Geometry check sheet. Reference: the model listing, model coordinates, mm. Face numbers are marked on the shaded views. A direction names the side the tool comes from. Round coordinates to 2 decimals unless told otherwise and drop trailing zeros. Loops run counter-clockwise (first coordinate to the right, second up) from the corner with the lowest first, then second, coordinate; pieces in that order, holes last.
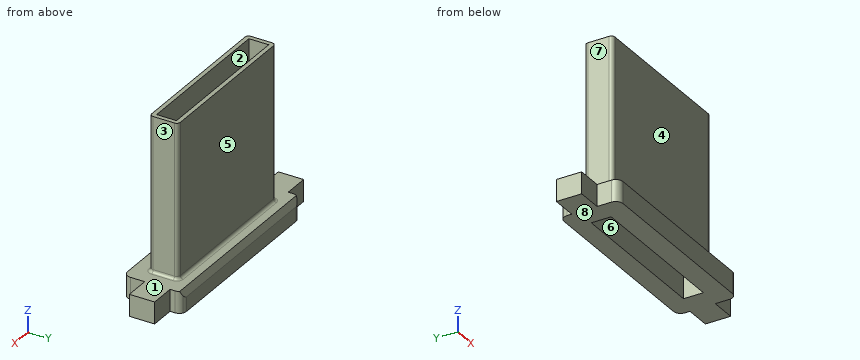
```python
from build123d import *

# Parameters (mm, degrees)
SKETCH1_W           = 53.8
SKETCH1_H           = 16.8
SKETCH1_W_2         = 42
SKETCH1_H_2         = 5.5
BOSS_EXTRUDE1_DEPTH = 27
SKETCH4_W           = 53.8
SKETCH4_H           = 16.8
SKETCH4_W_2         = 44.4
SKETCH4_H_2         = 7.9
CUT_EXTRUDE2_DEPTH  = 19.35
SKETCH2_W           = 7
SKETCH2_H           = 10
BOSS_EXTRUDE2_DEPTH = 6
SKETCH3_R           = 1.35
CUT_EXTRUDE1_DEPTH  = 8
CUT_EXTRUDE4_REACH  = 66.31
SKETCH7_W           = 53.8
SKETCH7_H           = 0.5
FILLET2_R           = 1
FILETE1_R           = 2
SKETCH5_W           = 53.8
SKETCH5_H           = 16.8
CUT_EXTRUDE3_DEPTH  = 1.65
CUT_EXTRUDE5_REACH  = 63.565
CUT_EXTRUDE6_REACH  = 64.931
BOSS_EXTRUDE3_START = -7
SKETCH10_R          = 1.35
BOSS_EXTRUDE3_DEPTH = 7
CUT_EXTRUDE7_DEPTH  = 1.65
SKETCH13_W          = 6
SKETCH13_H          = 16.8
CUT_EXTRUDE8_DEPTH  = 73.869901194
FILLET6_R           = 0.8
BOSS_EXTRUDE4_START = 3.9
SKETCH14_W          = 42
SKETCH14_H          = 5.5
BOSS_EXTRUDE4_DEPTH = 3.9


with BuildPart() as part:
    # Sketch1 → Boss-Extrude1 (new, symmetric)
    with BuildSketch(Plane.XY):
        Rectangle(SKETCH1_W, SKETCH1_H)
        Rectangle(SKETCH1_W_2, SKETCH1_H_2, mode=Mode.SUBTRACT)
    extrude(amount=BOSS_EXTRUDE1_DEPTH, both=True)

    # Sketch4 → Cut-Extrude2 (cut, symmetric)
    with BuildSketch(Plane.XY):
        Rectangle(SKETCH4_W, SKETCH4_H)
        Rectangle(SKETCH4_W_2, SKETCH4_H_2, mode=Mode.SUBTRACT)
    extrude(amount=CUT_EXTRUDE2_DEPTH, both=True, mode=Mode.SUBTRACT)

    # Sketch2 → Boss-Extrude2 (add)
    with BuildSketch(Plane(origin=(0, 0, 19.35), x_dir=(-1, 0, 0), z_dir=(0, 0, -1))):
        with Locations((-30.4, 2.55)):
            Rectangle(SKETCH2_W, SKETCH2_H)
        with Locations((30.4, 2.55)):
            Rectangle(SKETCH2_W, SKETCH2_H)
    boss_extrude2 = extrude(amount=-BOSS_EXTRUDE2_DEPTH)

    # Sketch3 → Cut-Extrude1 (cut)
    with BuildSketch(Plane.XZ.offset(2.45)):
        with Locations((-30.9, 22.35)):
            Circle(SKETCH3_R)
        with Locations((30.9, 22.35)):
            Circle(SKETCH3_R)
    cut_extrude1 = extrude(amount=-CUT_EXTRUDE1_DEPTH, mode=Mode.SUBTRACT)

    # Mirror8: Boss-Extrude2, Cut-Extrude1 across plane
    add(boss_extrude2.mirror(Plane.XY))
    add(cut_extrude1.mirror(Plane.XY), mode=Mode.SUBTRACT)

    # Sketch7 → Cut-Extrude4 (cut, up to next)
    with BuildSketch(Plane(origin=(0, 0, -27), x_dir=(-1, 0, 0), z_dir=(0, 0, -1)), mode=Mode.PRIVATE) as cut_extrude4_sk1:
        with Locations((0, 8.15)):
            Rectangle(SKETCH7_W, SKETCH7_H)
    cut_extrude4_tool1 = extrude(cut_extrude4_sk1.sketch, amount=-CUT_EXTRUDE4_REACH, mode=Mode.PRIVATE) & part.part
    add(cut_extrude4_tool1.solids().sort_by_distance((0, 8.15, -27))[0], mode=Mode.SUBTRACT)

    # Fillet2
    fillet2_edges = [part.edges().sort_by_distance(p)[0] for p in [
        (-22.2, -3.95, 0),
        (-22.2, 3.95, 0),
        (22.2, 3.95, 0),
        (22.2, -3.95, 0),
    ]]
    fillet(fillet2_edges, radius=FILLET2_R)

    # Filete1
    filete1_edges = [part.edges().sort_by_distance(p)[0] for p in [
        (-26.9, -8.4, -23.175),
        (26.9, -8.4, -23.175),
        (26.9, -8.4, 23.175),
        (-26.9, -8.4, 23.175),
        (26.9, 8.4, 23.175),
        (-26.9, 8.4, 23.175),
        (-26.9, 7.9, -23.175),
        (26.9, 7.9, -23.175),
    ]]
    fillet(filete1_edges, radius=FILETE1_R)

    # Sketch5 → Cut-Extrude3 (cut)
    with BuildSketch(Plane.XY.offset(27)):
        Rectangle(SKETCH5_W, SKETCH5_H)
    extrude(amount=-CUT_EXTRUDE3_DEPTH, mode=Mode.SUBTRACT)

    # Chamfer1
    # the kernel refuses this chamfer: 2, 0.890457371 mm, written as the material it takes off along each edge
    with BuildSketch(Plane(origin=(-37.34003391, 7.9, -19.35), x_dir=(0, -0.9968798599783938, 0.07893379991776824), z_dir=(1, 0, 0))) as chamfer1_piece_1:
        with BuildLine():
            Line((0.925885194, 0), (-0.196073774, 2.064046904))
            Line((-0.196073774, 2.064046904), (-0.235948969, 2.060889552))
            ThreePointArc((-0.235948969, 2.060889552), (-0.121693379, 1.030150311), (-0.039875194, -0.003157352))
            Line((-0.039875194, -0.003157352), (0.003157352, -0.039875194))
            ThreePointArc((0.003157352, -0.039875194), (0.463215564, -0.003447392), (0.929042546, -0.039875194))
            Line((0.929042546, -0.039875194), (0.925885194, 0))
        make_face()
    extrude(amount=74.680067819, mode=Mode.SUBTRACT)

    # Sketch8 → Cut-Extrude5 (cut, up to next)
    with BuildSketch(Plane(origin=(0, 0, -25.35), x_dir=(-1, 0, 0), z_dir=(0, 0, -1)), mode=Mode.PRIVATE) as cut_extrude5_sk1:
        with BuildLine():
            Line((-26.030265456, 7.55), (-33.9, 7.55))
            Line((-33.9, 7.55), (-33.9, 4.55))
            Line((-33.9, 4.55), (-26.9, 4.55))
            Line((-26.9, 4.55), (-26.9, 5.9))
            ThreePointArc((-26.9, 5.9), (-26.669255622, 6.832595595), (-26.030265456, 7.55))
        make_face()
    cut_extrude5_tool1 = extrude(cut_extrude5_sk1.sketch, amount=-CUT_EXTRUDE5_REACH, mode=Mode.PRIVATE) & part.part
    # Sketch8 → Cut-Extrude5 (cut, up to next)
    with BuildSketch(Plane(origin=(0, 0, -25.35), x_dir=(-1, 0, 0), z_dir=(0, 0, -1)), mode=Mode.PRIVATE) as cut_extrude5_sk2:
        with BuildLine():
            Line((26.9, 4.55), (26.9, 5.9))
            ThreePointArc((26.9, 5.9), (26.669255622, 6.832595595), (26.030265456, 7.55))
            Line((26.030265456, 7.55), (33.9, 7.55))
            Line((33.9, 7.55), (33.9, 4.55))
            Line((33.9, 4.55), (26.9, 4.55))
        make_face()
    cut_extrude5_tool2 = extrude(cut_extrude5_sk2.sketch, amount=-CUT_EXTRUDE5_REACH, mode=Mode.PRIVATE) & part.part
    add(cut_extrude5_tool1.solids().sort_by_distance((30.325305, 6.072078, -25.35))[0], mode=Mode.SUBTRACT)
    add(cut_extrude5_tool2.solids().sort_by_distance((-30.325305, 6.072078, -25.35))[0], mode=Mode.SUBTRACT)

    # Sketch9 → Cut-Extrude6 (cut, up to next)
    with BuildSketch(Plane.XY.offset(25.35), mode=Mode.PRIVATE) as cut_extrude6_sk1:
        Polygon((26.9, 5.9), (26.9, 7.55), (33.9, 7.55), (33.9, 4.55), (26.9, 4.55), align=None)
    cut_extrude6_tool1 = extrude(cut_extrude6_sk1.sketch, amount=-CUT_EXTRUDE6_REACH, mode=Mode.PRIVATE) & part.part
    # Sketch9 → Cut-Extrude6 (cut, up to next)
    with BuildSketch(Plane.XY.offset(25.35), mode=Mode.PRIVATE) as cut_extrude6_sk2:
        Polygon((-26.9, 5.9), (-26.9, 4.55), (-33.9, 4.55), (-33.9, 7.55), (-26.9, 7.55), align=None)
    cut_extrude6_tool2 = extrude(cut_extrude6_sk2.sketch, amount=-CUT_EXTRUDE6_REACH, mode=Mode.PRIVATE) & part.part
    add(cut_extrude6_tool1.solids().sort_by_distance((30.4, 6.05, 25.35))[0], mode=Mode.SUBTRACT)
    add(cut_extrude6_tool2.solids().sort_by_distance((-30.4, 6.05, 25.35))[0], mode=Mode.SUBTRACT)

    # Sketch10 → Boss-Extrude3 (add)
    with BuildSketch(Plane(origin=(0, 4.55, 0), x_dir=(1, 0, 0), z_dir=(0, 1, 0)).offset(BOSS_EXTRUDE3_START)):
        with Locations((30.9, -22.35)):
            Circle(SKETCH10_R)
        with Locations((-30.9, -22.35)):
            Circle(SKETCH10_R)
    boss_extrude3 = extrude(amount=BOSS_EXTRUDE3_DEPTH)

    # Mirror9: Boss-Extrude3 across plane
    add(boss_extrude3.mirror(Plane.XY))

    # Sketch11 → Cut-Extrude7 (cut)
    with BuildSketch(Plane(origin=(0, 0, -27), x_dir=(-1, 0, 0), z_dir=(0, 0, -1))):
        with BuildLine():
            Line((26.9, -6.4), (26.9, 5.9))
            ThreePointArc((26.9, 5.9), (26.314213562, 7.314213562), (24.9, 7.9))
            Line((24.9, 7.9), (-24.9, 7.9))
            ThreePointArc((-24.9, 7.9), (-26.314213562, 7.314213562), (-26.9, 5.9))
            Line((-26.9, 5.9), (-26.9, -6.4))
            ThreePointArc((-26.9, -6.4), (-26.314213562, -7.814213562), (-24.9, -8.4))
            Line((-24.9, -8.4), (24.9, -8.4))
            ThreePointArc((24.9, -8.4), (26.314213562, -7.814213562), (26.9, -6.4))
        make_face()
    extrude(amount=-CUT_EXTRUDE7_DEPTH, mode=Mode.SUBTRACT)

    # Sketch13 → Cut-Extrude8 (cut, through all)
    with BuildSketch(Plane.ZY.offset(33.9)):
        with Locations((22.35, 0)):
            Rectangle(SKETCH13_W, SKETCH13_H)
    extrude(amount=-CUT_EXTRUDE8_DEPTH, mode=Mode.SUBTRACT)

    # Fillet6
    fillet6_edges = [part.edges().sort_by_distance(p)[0] for p in [
        (-22.2, 0, -19.35),
        (0, -3.95, -19.35),
        (22.2, 0, -19.35),
        (0, 3.95, -19.35),
        (-21.907106781, -3.657106781, -19.35),
        (21.907106781, -3.657106781, -19.35),
        (21.907106781, 3.657106781, -19.35),
        (-21.907106781, 3.657106781, -19.35),
    ]]
    fillet(fillet6_edges, radius=FILLET6_R)

    # Sketch14 → Boss-Extrude4 (add)
    with BuildSketch(Plane.XY.offset(19.35).offset(BOSS_EXTRUDE4_START)):
        with BuildLine():
            Line((22.2, -2.95), (22.2, 2.95))
            ThreePointArc((22.2, 2.95), (21.907106781, 3.657106781), (21.2, 3.95))
            Line((21.2, 3.95), (-21.2, 3.95))
            ThreePointArc((-21.2, 3.95), (-21.907106781, 3.657106781), (-22.2, 2.95))
            Line((-22.2, 2.95), (-22.2, -2.95))
            ThreePointArc((-22.2, -2.95), (-21.907106781, -3.657106781), (-21.2, -3.95))
            Line((-21.2, -3.95), (21.2, -3.95))
            ThreePointArc((21.2, -3.95), (21.907106781, -3.657106781), (22.2, -2.95))
        make_face()
        Rectangle(SKETCH14_W, SKETCH14_H, mode=Mode.SUBTRACT)
    extrude(amount=-BOSS_EXTRUDE4_DEPTH)


solid = part.part
```
1) Mould release check, pull along X, two halves, no side actions. Record for the marked faces 6, 7 and 8: +X half, -X half, draft (parallel to the pull), parting line (faces both ways), or undercut.
Report:
face 6: undercut
face 7: -X half
face 8: draft
2) Scan lines: line 1 along X through (y, z) = (0.5, 5); line 2 along Y through (x, z) = (0.5, -2.5); line 3 along X through (y, z) = (-2, -20). Record each from-to range of solid material in increasing order.
Report:
line 1: x = -22.2 to -21, 21 to 22.2
line 2: y = -3.95 to -2.75, 2.75 to 3.95
line 3: x = -33.9 to -21, 21 to 33.9
3) Gauge pin test, flat ends, axial feed: pin 1 (6.5 mm diameter, centred on y = -1, z = -3, fed in from -X); pin 2 (3 mm diameter, centred on x = -29, z = -22, fed in from -Y); pin 3 (2 mm diameter, centred on x = 14, z = 7, fed in from +Y). Record the tip position at first contact, or that the pin passes through.
Report:
pin 1: stops at x = -22.2
pin 2: stops at y = -2.45
pin 3: stops at y = 3.95
4) Sectioned sample at B-B, the plane x = -6.5. Record the cut outline in (y, z), then the cut area to 3 significant figures.
Report:
outline: (-8.4, -25.35) - (-2.75, -25.35) - (-2.75, 23.25) - (-3.95, 23.25) - (-3.95, -18.55) arc R0.8 cw to (-4.75, -19.35) - (-8.4, -19.35) - close; (2.75, -25.35) - (7.9, -25.35) - (7.9, -21.35) - (7.01, -19.35) - (4.75, -19.35) arc R0.8 cw to (3.95, -18.55) - (3.95, 23.25) - (2.75, 23.25) - close
area: 166 mm2
5) Sectioned sample at A-A, the plane y = 1. Record the cut outline in (x, z), then the cut area to 3 significant figures.
Report:
outline: (-33.9, -25.35) - (-21, -25.35) - (-21, 23.25) - (-22.2, 23.25) - (-22.2, -18.55) arc R0.8 cw to (-23, -19.35) - (-33.9, -19.35) - close; (21, -25.35) - (33.9, -25.35) - (33.9, -19.35) - (23, -19.35) arc R0.8 cw to (22.2, -18.55) - (22.2, 23.25) - (21, 23.25) - close
area: 257 mm2
6) Access from +Z, -Z, +X, -X, +Y, -Y to the whole of each face (thin tool, end or side, straight path). Record for the marked faces 1, 2, 3, 4 and 5.
Report:
face 1: +Z
face 2: +Z, -Z
face 3: +Z, +X, +Y, -Y
face 4: +Z, +X, -X, -Y
face 5: +Z, +X, -X, +Y
7) Sectioned sample at C-C, the plane z = 9. Record the cut outline in (x, y).
Report:
outline: (-22.2, -2.95) arc R1 ccw to (-21.2, -3.95) - (21.2, -3.95) arc R1 ccw to (22.2, -2.95) - (22.2, 2.95) arc R1 ccw to (21.2, 3.95) - (-21.2, 3.95) arc R1 ccw to (-22.2, 2.95) - close; hole (-21, -2.75) - (21, -2.75) - (21, 2.75) - (-21, 2.75) - close
